The listing builds one solid part. Answer for the finished solid, in the listing's coordinates (mm). Face numbers are marked on the shaded views. A direction names the side the tool comes from. Coordinates: 2 decimals unless noted, no trailing zeros. Order: outer loops, then holes, each group sorted by start corner. A loop starts at its lowest first (then second) coordinate and runs counter-clockwise, first axis right, second up. Notation, with made-up numbers: (51, -1) - (110, -1) arc R21 cw to (110, 25) - close; hole circle Ø5 at (-10, 66.5). An arc over 180 degrees is marked (long way). Use one line per item in the form item = value. Start each with the question number.
Item 1: Section D-D, the plane x = -19.5 is taken. Write down the section's boundary in (y, z).
Item 2: A tool of negligible diameter and unlimited length cuts with its end or side. For the marked faces 1, 2 and 3, from which of +Z, -Z, +X, -X, +Y, -Y can it reach the whole face along a straight path? Write none if from no direction.
Item 3: Section A-A, the plane y = 0 is taken. Write down the section's boundary in (x, z).
Item 4: Section B-B, the plane z = -3.5 is taken. Write down the section's boundary in (x, y), and give its area (3 significant figures).
Item 5: Section C-C, the plane y = -12.5 is taken. Write down the section's boundary in (x, z), and give its area (3 significant figures).
Item 6: Each of these flat-tipped pins is pushed along its axis until it touches: pin 1 Ø6 at (x, y) = (-21.5, 7) entering from -Z; pin 2 Ø5 at (y, z) = (12.5, -21.65) entering from +X; pin 3 Ø1 at (x, y) = (-17, -5.5) entering from +Z. Where does it stop, or does it pass through?
Item 7: The mould has two halves that part along Y. Classify the marked faces 4, 5, 6 and 7: released by +Y, released by -Y, zero draft, split by the parting line, or undercut.
Item 8: Consider line 1 along Z through (x, y) = (-37, 12); line 2 along Z through (x, y) = (-33.75, -12.5); line 3 along X through (y, z) = (-2, 22). Determine where each line is inside the solid, lowest interval first. Write a range as [from, to].
from build123d import *

# Parameters (mm, degrees)
F0_R     = 30
F1_DEPTH = 40
F2_R     = 30
F2_R_2   = 20
F3_DEPTH = 30
F5_DEPTH = 40.001
F6_R     = 2
F7_DEPTH = 40.001
F8_R     = 10
F9_DEPTH = 40.001


with BuildPart() as f1:
    # F0 (on Right) → F1 (new body)
    with BuildSketch(Plane.YZ):
        Circle(F0_R)
    extrude(amount=-F1_DEPTH)

    # F2 (on face) → F3 (cut)
    with BuildSketch(Plane.YZ):
        Circle(F2_R)
        Circle(F2_R_2, mode=Mode.SUBTRACT)
    extrude(amount=-F3_DEPTH, mode=Mode.SUBTRACT)

    # F4 (on face) → F5 (cut, through all)
    with BuildSketch(Plane(origin=(-40, 0, 0), x_dir=(0, -1, 0), z_dir=(-1, 0, 0))):
        with BuildLine():
            Line((-20, -22.36068), (-20, 22.36068))
            ThreePointArc((-20, 22.36068), (-30, 0), (-20, -22.36068))
        make_face()
        with BuildLine():
            ThreePointArc((30, 0), (27.386128, 12.247449), (20, 22.36068))
            Line((20, 22.36068), (20, -22.36068))
            ThreePointArc((20, -22.36068), (27.386128, -12.247449), (30, 0))
        make_face()
    extrude(amount=-F5_DEPTH, mode=Mode.SUBTRACT)

    # F6 (on face) → F7 (cut, through all)
    with BuildSketch(Plane(origin=(-40, 0, 0), x_dir=(0, -1, 0), z_dir=(-1, 0, 0))):
        with Locations((12.5, 21.650635)):
            Circle(F6_R)
        with Locations((-12.5, 21.650635)):
            Circle(F6_R)
        with Locations((12.5, -21.650635)):
            Circle(F6_R)
        with Locations((-12.5, -21.650635)):
            Circle(F6_R)
    extrude(amount=-F7_DEPTH, mode=Mode.SUBTRACT)

    # F8 (on face) → F9 (cut, through all)
    with BuildSketch(Plane(origin=(-40, 0, 0), x_dir=(0, -1, 0), z_dir=(-1, 0, 0))):
        Circle(F8_R)
    extrude(amount=-F9_DEPTH, mode=Mode.SUBTRACT)


solid = f1.part
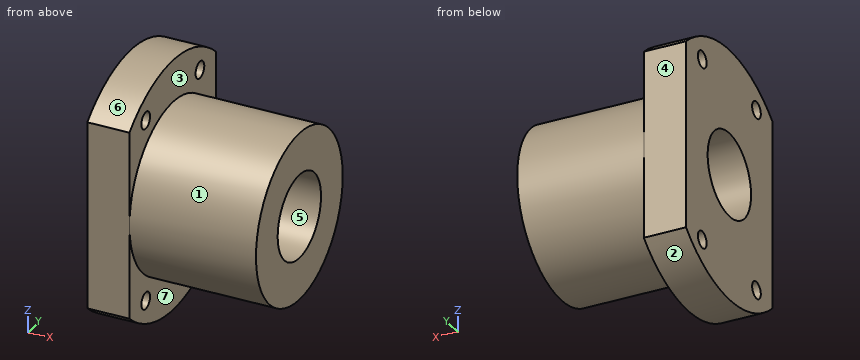
Response:
q1.outline = circle Ø40 at (0, 0); hole circle Ø20 at (0, 0)
q2.face_1 = +X
q2.face_2 = -Z, +X, -X
q2.face_3 = +Z, +X
q3.outline = (-40, -30) - (-30, -30) - (-30, -20) - (0, -20) - (0, -10) - (-40, -10) - close; (-40, 10) - (0, 10) - (0, 20) - (-30, 20) - (-30, 30) - (-40, 30) - close
q4.outline = (-40, -20) - (-30, -20) - (-30, -19.69) - (0, -19.69) - (0, -9.37) - (-40, -9.37) - close; (-40, 9.37) - (0, 9.37) - (0, 19.69) - (-30, 19.69) - (-30, 20) - (-40, 20) - close
q4.area = 832 mm2
q5.outline = (-40, -27.27) - (-30, -27.27) - (-30, -23.65) - (-40, -23.65) - close; (-40, -19.65) - (-30, -19.65) - (-30, -15.61) - (0, -15.61) - (0, 15.61) - (-30, 15.61) - (-30, 19.65) - (-40, 19.65) - close; (-40, 23.65) - (-30, 23.65) - (-30, 27.27) - (-40, 27.27) - close
q5.area = 1,400 mm2
q6.pin_1 = -19.6
q6.pin_2 = -30
q6.pin_3 = 19.36
q7.face_4 = released by +Y
q7.face_5 = undercut
q7.face_6 = split by the parting line
q7.face_7 = zero draft
q8.line_1 = [-27.5, -23.59], [-19.71, 19.71], [23.59, 27.5]
q8.line_2 = [-27.27, -23.65], [-19.65, 19.65], [23.65, 27.27]
q8.line_3 = [-40, -30]
